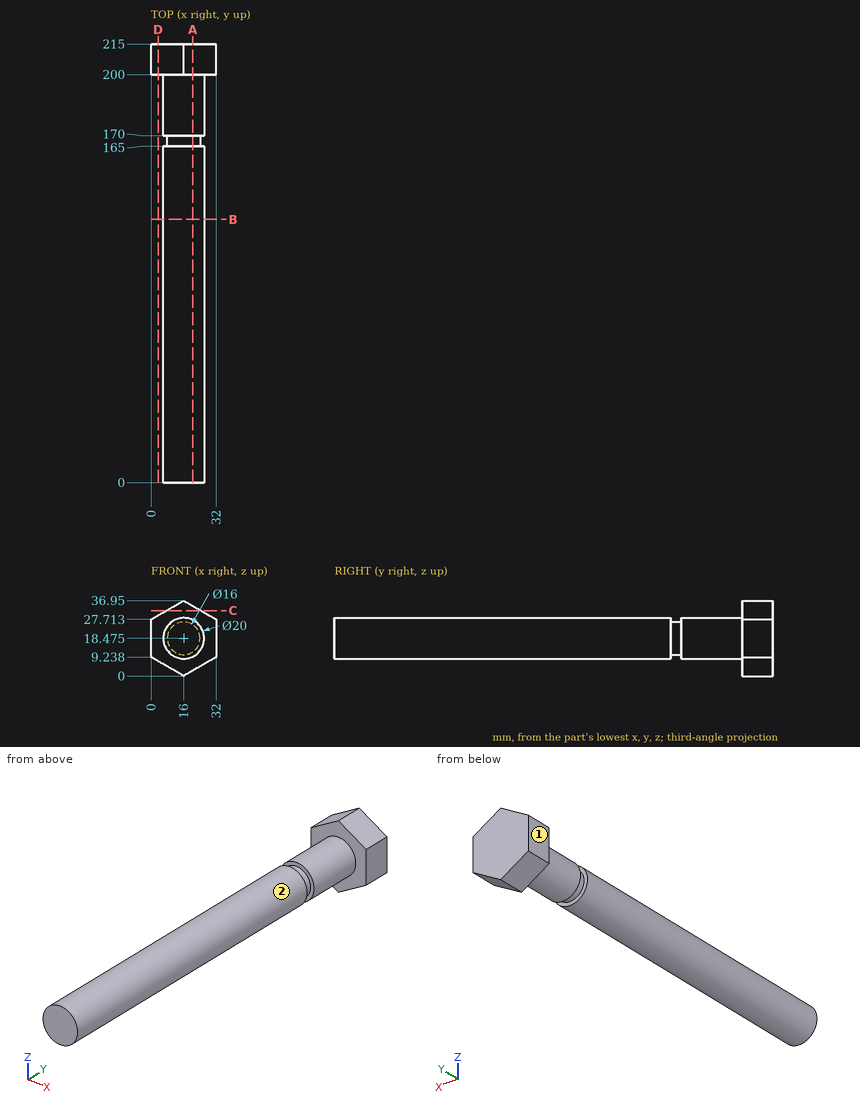
Can you work these out from the drawing? Everything is in mm from the part's minimum corner. A direction names the side the tool comes from. Round coordinates to 2 decimals unless told otherwise and drop trailing zeros. Loops run counter-clockwise (first coordinate to the right, second up) from the corner with the lowest first, then second, coordinate; pieces in that order, holes last. Notation, with made-up numbers: (73.5, 6.5) - (85.5, 6.5) arc R23 ccw to (85.5, 44.5) - close; hole circle Ø3 at (54.25, -25.5). An arc over 180 degrees is marked (long way). Answer in a Markdown table with one row per item. Add a question column.
Q1. Which directions (+Z, -Z, +X, -X, +Y, -Y) give clear straight access to the entire face, cutting with the end or side of a thin tool? Please do the marked faces 1 and 2.
Q2. I want a section at A-A on x = 20.5. List the corners of the cut face in (y, z) for me (1 decimal).
Q3. I want a section at C-C on z = 32. List the corners of the cut face in (x, y) for me (1 decimal), and give its area (3 significant figures).
Q4. For pin 1 Ø10 at (y, z) = (63, 12.5) entering from -X; pin 2 Ø12 at (y, z) = (123.5, 22) entering from +X; pin 3 Ø12 at (y, z) = (75.5, 25.5) entering from -X; pin 4 Ø1 at (x, y) = (4, 30) entering from -Z, each with a flat end and sliding along its axis, tell me the tip position at first contact or that it passes through.
Q5. I want a section at B-B on y = 129. List the corners of the cut face in (x, z) for me (1 decimal).
Q6. I want a section at D-D on x = 3.5. List the corners of the cut face in (y, z) for me.
Q7. I need wall thicknesses on L1, parallel to Z at x = 10, y = 139 (1 decimal); L2, parallel to Y at x = 29.5, z = 13; L3, parallel to Y at x = 20, z = 11. Which ranges of each line are inside material? Lowest first, please.
A:
| question | item | result |
|---|---|---|
| 1 | face 1 | +Z, -Z, -X, +Y, -Y |
| 1 | face 2 | -Y |
| 2 | outline | (0, 9.5) - (165, 9.5) - (165, 11.9) - (170, 11.9) - (170, 9.5) - (200, 9.5) - (200, 2.6) - (215, 2.6) - (215, 34.4) - (200, 34.4) - (200, 27.4) - (170, 27.4) - (170, 25.1) - (165, 25.1) - (165, 27.4) - (0, 27.4) - close |
| 3 | outline | (7.4, 200) - (24.6, 200) - (24.6, 215) - (7.4, 215) - close |
| 3 | area | 257 mm^2 |
| 4 | pin 1 | x = 6.05 |
| 4 | pin 2 | x = 26 |
| 4 | pin 3 | x = 6.05 |
| 4 | pin 4 | through |
| 5 | outline | circle Ø20 at (16, 18.5) |
| 6 | outline | (200, 7.22) - (215, 7.22) - (215, 29.73) - (200, 29.73) - close |
| 7 | L1 | 10.5 to 26.5 |
| 7 | L2 | 200 to 215 |
| 7 | L3 | 0 to 165, 170 to 215 |
